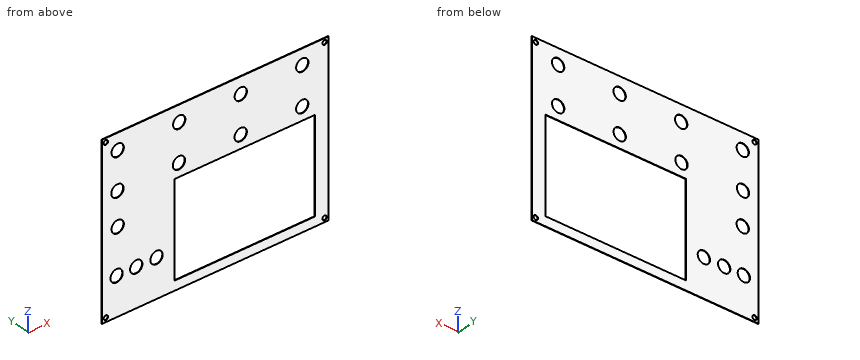
```python
from build123d import *

# Parameters (mm, degrees)
SKETCH1_W           = 128.872
SKETCH1_H           = 96.012
SKETCH1_R           = 1.25
SKETCH1_R_2         = 3.5
SKETCH1_W_2         = 80
SKETCH1_H_2         = 53
BOSS_EXTRUDE1_DEPTH = 0.3


with BuildPart() as part:
    # Sketch1 → Boss-Extrude1 (new body)
    with BuildSketch(Plane(origin=(0, 0, 0), x_dir=(1, 0, 0), z_dir=(0, 1, 0))):
        with Locations((62.15, 45.72)):
            Rectangle(SKETCH1_W, SKETCH1_H)
        with Locations(Location((0, 91.44, 0), (0, 0, 270))):
            Circle(SKETCH1_R, mode=Mode.SUBTRACT)
        with Locations(Location((124.3, 91.44, 0), (0, 0, 270))):
            Circle(SKETCH1_R, mode=Mode.SUBTRACT)
        with Locations(Location((0, 0, 0), (0, 0, 270))):
            Circle(SKETCH1_R, mode=Mode.SUBTRACT)
        with Locations(Location((124.3, 0, 0), (0, 0, 270))):
            Circle(SKETCH1_R, mode=Mode.SUBTRACT)
        with Locations(Location((6.731, 6.881, 0), (0, 0, 270))):
            Circle(SKETCH1_R_2, mode=Mode.SUBTRACT)
        with Locations(Location((41.697, 6.881, 0), (0, 0, 270))):
            Circle(SKETCH1_R_2, mode=Mode.SUBTRACT)
        with Locations(Location((76.663, 6.881, 0), (0, 0, 270))):
            Circle(SKETCH1_R_2, mode=Mode.SUBTRACT)
        with Locations(Location((111.63, 6.44, 0), (0, 0, 270))):
            Circle(SKETCH1_R_2, mode=Mode.SUBTRACT)
        with Locations(Location((6.73, 46.754, 0), (0, 0, 270))):
            Circle(SKETCH1_R_2, mode=Mode.SUBTRACT)
        with Locations(Location((6.568, 28.023, 0), (0, 0, 270))):
            Circle(SKETCH1_R_2, mode=Mode.SUBTRACT)
        with Locations(Location((41.524, 28.023, 0), (0, 0, 270))):
            Circle(SKETCH1_R_2, mode=Mode.SUBTRACT)
        with Locations(Location((76.645, 28.023, 0), (0, 0, 270))):
            Circle(SKETCH1_R_2, mode=Mode.SUBTRACT)
        with Locations(Location((111.601, 28.023, 0), (0, 0, 270))):
            Circle(SKETCH1_R_2, mode=Mode.SUBTRACT)
        with Locations(Location((6.096, 72.09, 0), (0, 0, 270))):
            Circle(SKETCH1_R_2, mode=Mode.SUBTRACT)
        with Locations(Location((17.272, 72.09, 0), (0, 0, 270))):
            Circle(SKETCH1_R_2, mode=Mode.SUBTRACT)
        with Locations(Location((28.83, 72.09, 0), (0, 0, 270))):
            Circle(SKETCH1_R_2, mode=Mode.SUBTRACT)
        with Locations((78.875410923, 61.951987271)):
            Rectangle(SKETCH1_W_2, SKETCH1_H_2, mode=Mode.SUBTRACT)
    extrude(amount=BOSS_EXTRUDE1_DEPTH)


solid = part.part
```
Here's how the part is built. I have some questions about the finished solid (model axes, mm). Round coordinates to 2 decimals unless told otherwise and drop trailing zeros. Write each loop counter-clockwise with the first axis right and the second up, starting at its lowest first coordinate (ties: lowest second). Pieces come first, ordered by that corner, then holes.
Q1. If we section it at D-D on y = 0.2: Give the number of separate pieces and of enclosed holes in the cut face, plus the area to 3 significant figures.
Q2. If we section it at A-A on x = 28.83: Write out the boundary of the cut face in (y, z), plus the area to 3 significant figures.
Q3. If we section it at C-C on x = 75: Write out the boundary of the cut face in (y, z), plus the area to 3 significant figures.
Q4. Please list where these lines run through material, in increasing order: probe 1 along X at (y, z) = (0.2, -91.44); probe 2 along Z at (x, y) = (124.3, 0.2); probe 3 along Z at (x, y) = (75, 0.15).
Q5. If we section it at B-B on z = -72.09: Write out the boundary of the cut face in (x, y), plus the area to 3 significant figures.
Q6. Will these pins go through, and if not, where does the flat tip stop? P1, Ø9, axis at x = 41.524, z = -28.023, coming from the +Y side; P2, Ø4, axis at x = 28.83, z = -72.09, coming from the +Y side.
Answer below:
1. separate pieces: 1
1. enclosed holes: 17
1. area: 7,650 mm2
2. outline: (0, -93.73) - (0.3, -93.73) - (0.3, -75.59) - (0, -75.59) - close; (0, -68.59) - (0.3, -68.59) - (0.3, 2.29) - (0, 2.29) - close
2. area: 26.7 mm2
3. outline: (0, -93.73) - (0.3, -93.73) - (0.3, -88.45) - (0, -88.45) - close; (0, -35.45) - (0.3, -35.45) - (0.3, -31.11) - (0, -31.11) - close; (0, -24.93) - (0.3, -24.93) - (0.3, -9.96) - (0, -9.96) - close; (0, -3.8) - (0.3, -3.8) - (0.3, 2.29) - (0, 2.29) - close
3. area: 9.20 mm2
4. probe 1: x = -2.29 to -1.25, 1.25 to 123.05, 125.55 to 126.59
4. probe 2: z = -93.73 to -92.69, -90.19 to -1.25, 1.25 to 2.29
4. probe 3: z = -93.73 to -88.45, -35.45 to -31.11, -24.93 to -9.96, -3.8 to 2.29
5. outline: (-2.29, 0) - (2.6, 0) - (2.6, 0.3) - (-2.29, 0.3) - close; (9.6, 0) - (13.77, 0) - (13.77, 0.3) - (9.6, 0.3) - close; (20.77, 0) - (25.33, 0) - (25.33, 0.3) - (20.77, 0.3) - close; (32.33, 0) - (38.88, 0) - (38.88, 0.3) - (32.33, 0.3) - close; (118.88, 0) - (126.59, 0) - (126.59, 0.3) - (118.88, 0.3) - close
5. area: 8.36 mm2
6. P1: stops at y = 0.3
6. P2: passes through
